Can you work these out from the drawing? Everything is in mm from the part's minimum corner. A direction names the side the tool comes from. Round coordinates to 2 decimals unless told otherwise and drop trailing zeros. Order: outer loops, then holes, each group sorted by start corner. A loop starts at its lowest first (then second) coordinate and runs counter-clockwise, first axis right, second up. Notation, with made-up numbers: (76.5, 69.5) - (115.5, 69.5) arc R20 ccw to (115.5, 93.5) - close; hole circle Ø3 at (9.5, 34). An arc over 180 degrees is marked (long way). Answer as a JSON object with one key per item and string values.
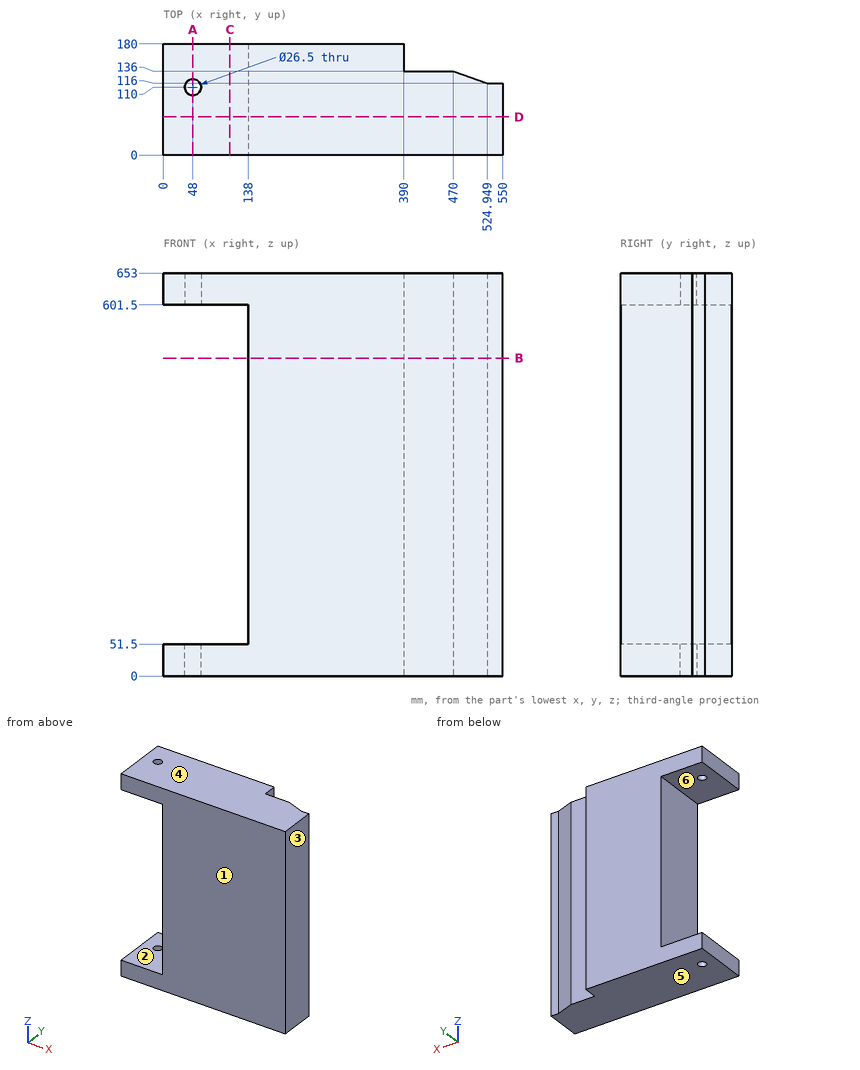
1. Thinking about a two-plate mould opening in Z: for the marked faces 3, 4, 5 and 6, which applies, pulls with the +Z half, pulls with the -Z half, needs draft (parallel to the pull), parting line crosses it, or undercut?
Responses:
{"face 3": "needs draft", "face 4": "pulls with the +Z half", "face 5": "pulls with the -Z half", "face 6": "undercut"}
2. For the marked faces 1 and 2, which set-ups out of +Z, -Z, +X, -X, +Y, -Y let a thin tool reach every point of the face, with its end or its side?
Responses:
{"face 1": "+Z, -Z, +X, -X, -Y", "face 2": "-X, +Y, -Y"}
3. Imagine slicing it at B-B (z = 515). List the corners of the cut face in (x, y) for me, plus the area to 3 significant figures.
Responses:
{"outline": "(138, 0) - (550, 0) - (550, 116) - (524.95, 116) - (470, 136) - (390, 136) - (390, 180) - (138, 180) - close", "area": "66,100 mm2"}
4. Imagine slicing it at D-D (y = 62). List the corners of the cut face in (x, z) for me.
Responses:
{"outline": "(0, 0) - (550, 0) - (550, 653) - (0, 653) - (0, 601.5) - (138, 601.5) - (138, 51.5) - (0, 51.5) - close"}
5. Imagine slicing it at C-C (x = 108). List the corners of the cut face in (y, z) for me.
Responses:
{"outline": "(0, 0) - (180, 0) - (180, 51.5) - (0, 51.5) - close; (0, 601.5) - (180, 601.5) - (180, 653) - (0, 653) - close"}
6. Imagine slicing it at A-A (x = 48). List the corners of the cut face in (y, z) for me.
Responses:
{"outline": "(0, 0) - (96.75, 0) - (96.75, 51.5) - (0, 51.5) - close; (0, 601.5) - (96.75, 601.5) - (96.75, 653) - (0, 653) - close; (123.25, 0) - (180, 0) - (180, 51.5) - (123.25, 51.5) - close; (123.25, 601.5) - (180, 601.5) - (180, 653) - (123.25, 653) - close"}
7. If I drill on L1, parallel to X at y = 110, z = 21; L2, parallel to Z at x = 115.5, y = 98; L3, parallel to X at y = 26, z = 466.5, over which ranges is the centre line in solid material (lowest first)? Write a range as [from, to].
Responses:
{"L1": "[0, 34.75], [61.25, 550]", "L2": "[0, 51.5], [601.5, 653]", "L3": "[138, 550]"}
8. For P1, Ø10, axis at x = 477.5, z = 199, coming from the +Y side, with a flat end and sliding along its axis, tell me the tip position at first contact or that it passes through.
Responses:
{"P1": "y = 135.09"}
